Geometry: see drawing. Coordinates: mm, zero at the bounding-box minimum. A direction names the side the tool comes from. Coordinates: 2 decimals unless noted, no trailing zeros. Loops run counter-clockwise (first coordinate to the right, second up) from the corner with the lowest first, then second, coordinate; pieces in that order, holes last.
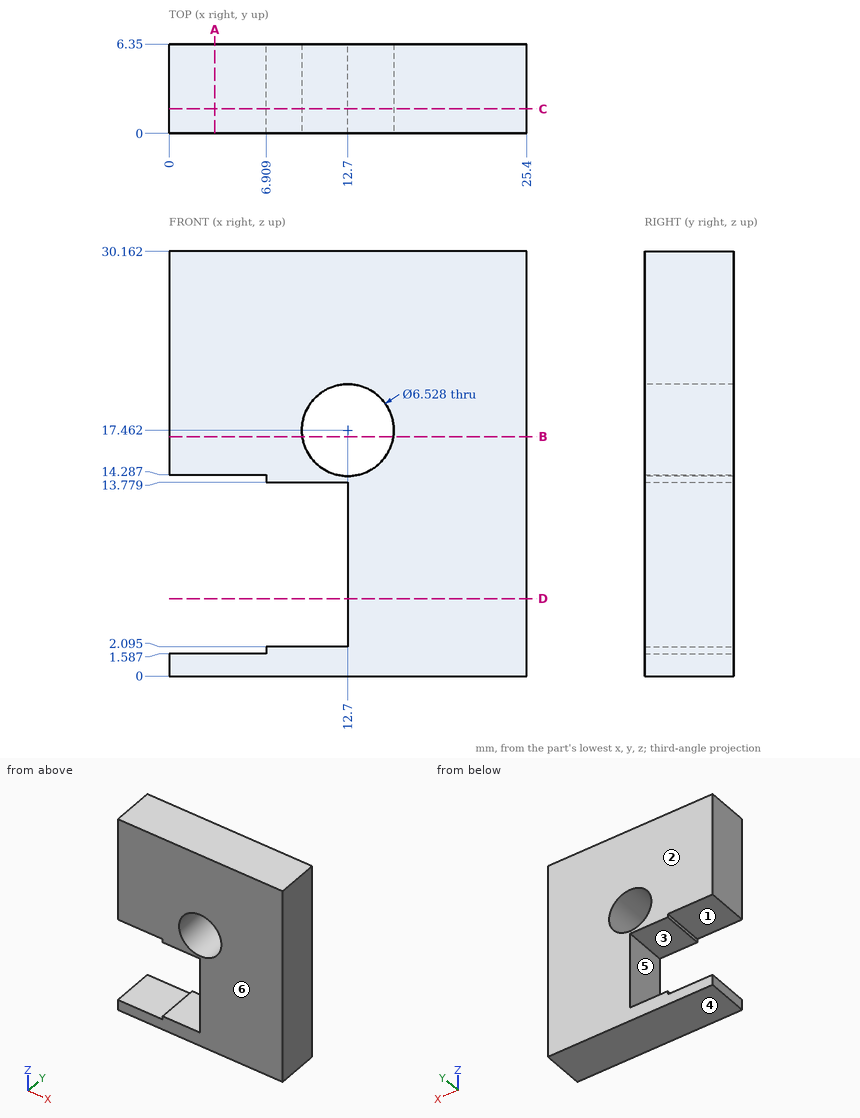
Item 1: Section query A-A (x = 3.25). Output: boundary loops of the cut face in (y, z), then the cut area to 3 significant figures.
Result:
outline: (0, 0) - (6.35, 0) - (6.35, 1.59) - (0, 1.59) - close; (0, 14.29) - (6.35, 14.29) - (6.35, 30.16) - (0, 30.16) - close
area: 111 mm2
Item 2: Section query B-B (z = 17). Output: boundary loops of the cut face in (x, y).
Result:
outline: (0, 0) - (9.47, 0) - (9.47, 6.35) - (0, 6.35) - close; (15.93, 0) - (25.4, 0) - (25.4, 6.35) - (15.93, 6.35) - close
Item 3: Section query D-D (z = 5.5). Output: boundary loops of the cut face in (x, y).
Result:
outline: (12.7, 0) - (25.4, 0) - (25.4, 6.35) - (12.7, 6.35) - close
Item 4: Mould query, pull axis Z, two halves, no side actions, for the marked faces 1, 2, 3 and 4. Classes: +Z half, -Z half, draft (parallel to the pull), parting line (faces both ways), or undercut.
Result:
face 1: undercut
face 2: draft
face 3: undercut
face 4: -Z half
Item 5: Line query: L1, parallel to Z at x = 3, y = 4.75; L2, parallel to Z at x = 11.5, y = 3.5 (1 decimal); L3, parallel to Z at x = 12.75, y = 6 (1 decimal). Output: solid intervals per line, ascending.
Result:
L1: z = 0 to 1.59, 14.29 to 30.16
L2: z = 0 to 2.1, 13.8 to 14.4, 20.5 to 30.2
L3: z = 0 to 14.2, 20.7 to 30.2
Item 6: Reachability of the marked faces 5 and 6 from +Z, -Z, +X, -X, +Y, -Y: full face, straight path, thin tool, end or side. Return the list, or none.
Result:
face 5: -X, +Y, -Y
face 6: +Z, -Z, +X, -X, -Y
Item 7: Contact query for flat-ended pins moving along their axis: P1, Ø2, axis at y = 2.5, z = 15, coming from the -X side; P2, Ø1.5, axis at y = 5.5, z = 11, coming from the -X side. Output: stop coordinate, or through.
Result:
P1: stops at x = 0
P2: stops at x = 12.7
Item 8: Section query C-C (y = 1.75). Output: boundary loops of the cut face in (x, z) (1 decimal), then the cut area to 3 significant figures.
Result:
outline: (0, 0) - (25.4, 0) - (25.4, 30.2) - (0, 30.2) - (0, 14.3) - (6.9, 14.3) - (6.9, 13.8) - (12.7, 13.8) - (12.7, 2.1) - (6.9, 2.1) - (6.9, 1.6) - (0, 1.6) - close; hole circle Ø6.5 at (12.7, 17.5)
area: 577 mm2
